Verification items for the finished model (mm, model axes). Round coordinates to 2 decimals unless told otherwise and drop trailing zeros. Loops run counter-clockwise (first coordinate to the right, second up) from the corner with the lowest first, then second, coordinate; pieces in that order, holes last. Notation, with made-up numbers: (25.25, 25.25) -> (29.25, 25.25) arc R28 cw to (29.25, 43.25) -> close; hole circle Ø5 at (48.25, 39.5). An arc over 180 degrees is marked (long way). Write item = value, one per line. Start each with the question number.
```python
from build123d import *

# Parameters (mm, degrees)
SKETCH1_W               = 22
SKETCH1_H               = 22
EXTRUDE1_DEPTH          = 40
EXTRUDE2_DEPTH          = 12
EXTRUDE2_DEPTH_BACK     = 12
SKETCH3_R               = 5
EXTRUDE3_DEPTH          = 11
EXTRUDE3_DEPTH_BACK     = 11
F_5_8_18_TAPPED_HOLE1_D = 14.68374


with BuildPart() as part:
    # Sketch1 → Extrude1 (new body)
    with BuildSketch(Plane.XY):
        Rectangle(SKETCH1_W, SKETCH1_H)
    extrude(amount=EXTRUDE1_DEPTH)

    # Sketch2 → Extrude2 (cut, two sides)
    with BuildSketch(Plane(origin=(0, 0, 0), x_dir=(0, 0, -1), z_dir=(1, 0, 0))) as extrude2_sk:
        with BuildLine():
            Line((-11, -10), (-49.420419849, -10))
            Line((-49.420419849, -10), (-49.420419849, -16.887372299))
            Line((-49.420419849, -16.887372299), (-11, -16.887372299))
            Line((-11, -16.887372299), (8.616222101, -16.887372299))
            Line((8.616222101, -16.887372299), (8.616222101, 23.046405641))
            Line((8.616222101, 23.046405641), (-11, 23.046405641))
            Line((-11, 23.046405641), (-49.420419849, 23.046405641))
            Line((-49.420419849, 23.046405641), (-49.420419849, 10))
            Line((-49.420419849, 10), (-11, 10))
            ThreePointArc((-11, 10), (-1, 0), (-11, -10))
        make_face()
    extrude(amount=EXTRUDE2_DEPTH, mode=Mode.SUBTRACT)
    extrude(extrude2_sk.sketch, amount=-EXTRUDE2_DEPTH_BACK, mode=Mode.SUBTRACT)

    # Sketch3 → Extrude3 (cut, two sides)
    with BuildSketch(Plane(origin=(0, 0, 0), x_dir=(1, 0, 0), z_dir=(0, 1, 0))) as extrude3_sk:
        with Locations((0, -25)):
            Circle(SKETCH3_R)
        with BuildLine():
            Line((-18.844545226, 6.847618329), (-7.5, 6.847618329))
            Line((-7.5, 6.847618329), (-7.5, -25))
            ThreePointArc((-7.5, -25), (0, -32.5), (7.5, -25))
            Line((7.5, -25), (7.5, 6.847618329))
            Line((7.5, 6.847618329), (23.30888992, 6.847618329))
            Line((23.30888992, 6.847618329), (23.30888992, -44.330247861))
            Line((23.30888992, -44.330247861), (-18.844545226, -44.330247861))
            Line((-18.844545226, -44.330247861), (-18.844545226, 6.847618329))
        make_face()
    extrude(amount=EXTRUDE3_DEPTH, mode=Mode.SUBTRACT)
    extrude(extrude3_sk.sketch, amount=-EXTRUDE3_DEPTH_BACK, mode=Mode.SUBTRACT)

    # 5/8-18 Tapped Hole1 (through all)
    with Locations(Plane(origin=(7.5, 0, 0), x_dir=(0, 0, -1), z_dir=(1, 0, 0))):
        with Locations((-11, 0)):
            Hole(F_5_8_18_TAPPED_HOLE1_D / 2)


solid = part.part
```
(1) Section check C-C on z = 23.5. Enter the section's corners in (x, y).
(2) Scan lines: line 1 (Z direction, x = 0, y = -0.25); line 2 (Z direction, x = 0, y = -1.25); line 3 (Y direction, x = -2.75, z = 11). Record each from-to range of solid material in increasing order. Write a range as [from, to].
(3) Depth check by flat-ended pin: pin 1 Ø2 at (x, y) = (-5, 3.5) entering from -Z; pin 2 Ø5 at (x, y) = (-4, -4) entering from +Z; pin 3 Ø5 at (x, z) = (2, 7) entering from +Y. Enter the tip coordinate at first touch or a pass-through.
(4) Section check D-D on x = -6.25. Enter the section's corners in (y, z), then the cut area to 3 significant figures.
(5) Section check B-B on y = 0. Enter the section's corners in (x, z), then the cut area to 3 significant figures.
(6) Draft check along Y on faces 1 (the flat face through (0, -10, 19)), 2 (the cylindrical face through (0, 0, 1)), 3 (the cylindrical face through (-0.105, -2.812, 17.782)). Enter one of: +Y half, -Y half, draft (parallel to the pull), parting line (faces both ways), or undercut.
(7) Section check A-A on x = 0. Enter the section's corners in (y, z).
Computed values:
q1.outline = (-7.5, -10) -> (-4.77, -10) -> (-4.77, 10) -> (-7.5, 10) -> close; (4.77, -10) -> (7.5, -10) -> (7.5, 10) -> (4.77, 10) -> close
q2.line_1 = [1, 3.66], [18.34, 20], [30, 32.5]
q2.line_2 = [1.08, 3.77], [18.23, 20], [30, 32.5]
q2.line_3 = [-10, -7.34], [7.34, 10]
q3.pin_1 = 1.32
q3.pin_2 = 32.35
q3.pin_3 = 9.89
q4.outline = (-10, 11) arc R10 ccw to (10, 11) -> (10, 29.15) -> (-10, 29.15) -> close; hole circle Ø14.68 at (0, 11)
q4.area = 351 mm²
q5.outline = (-7.5, 1) -> (7.5, 1) -> (7.5, 3.66) -> (-7.5, 3.66) -> close; (-7.5, 18.34) -> (7.5, 18.34) -> (7.5, 25) arc R7.5 ccw to (-7.5, 25) -> close; hole circle Ø10 at (0, 25)
q5.area = 150 mm²
q6.face_1 = -Y half
q6.face_2 = parting line
q6.face_3 = undercut
q7.outline = (-10, 11) arc R10 ccw to (10, 11) -> (10, 20) -> (-10, 20) -> close; (-10, 30) -> (10, 30) -> (10, 32.5) -> (-10, 32.5) -> close; hole circle Ø14.68 at (0, 11)
